```python
from build123d import *

# Parameters (mm, degrees)
SKETCH1_R           = 6.35
BOSS_EXTRUDE1_DEPTH = 254
SKETCH2_R           = 5.08
BOSS_EXTRUDE2_DEPTH = 203.2
SKETCH3_R           = 3.81
BOSS_EXTRUDE3_DEPTH = 152.4
SKETCH4_R           = 5.08
BOSS_EXTRUDE4_DEPTH = 7.62
FILLET1_R           = 2.54


with BuildPart() as part:
    # Sketch1 → Boss-Extrude1 (new body)
    with BuildSketch(Plane(origin=(0, 0, 0), x_dir=(1, 0, 0), z_dir=(0, 1, 0))):
        with Locations(Location((0, 0, 0), (0, 0, 270))):
            Circle(SKETCH1_R)
    extrude(amount=BOSS_EXTRUDE1_DEPTH)

    # Sketch2 → Boss-Extrude2 (add)
    with BuildSketch(Plane(origin=(0, 254, 0), x_dir=(1, 0, 0), z_dir=(0, 1, 0))):
        with Locations(Location((0, 0, 0), (0, 0, 270))):
            Circle(SKETCH2_R)
    extrude(amount=BOSS_EXTRUDE2_DEPTH)

    # Sketch3 → Boss-Extrude3 (add)
    with BuildSketch(Plane(origin=(0, 457.2, 0), x_dir=(1, 0, 0), z_dir=(0, 1, 0))):
        with Locations(Location((0, 0, 0), (0, 0, 90))):
            Circle(SKETCH3_R)
    extrude(amount=BOSS_EXTRUDE3_DEPTH)

    # Sketch4 → Boss-Extrude4 (add)
    with BuildSketch(Plane(origin=(0, 609.6, 0), x_dir=(1, 0, 0), z_dir=(0, 1, 0))):
        with Locations(Location((0, 0, 0), (0, 0, 270))):
            Circle(SKETCH4_R)
    extrude(amount=BOSS_EXTRUDE4_DEPTH)

    # Fillet1
    # the kernel refuses this fillet: 2.54 mm, written as the material it takes off along each edge
    with BuildSketch(Plane(origin=(0, 609.6, 0), x_dir=(0, 0, 1), z_dir=(-1, 0, 0))) as fillet1_piece_1:
        with BuildLine():
            CenterArc((2.54, 2.199704526), FILLET1_R, 300, 60)
            Line((3.81, 0), (3.8354, -0.043994091))
            ThreePointArc((3.8354, -0.043994091), (4.445, -0.0508), (5.08, -0.0508))
            Line((5.08, -0.0508), (5.1308, 0))
            Line((5.1308, 0), (5.1308, 2.199704526))
            Line((5.1308, 2.199704526), (5.08, 2.199704526))
        make_face()
    revolve(axis=Axis((0, 609.6, 0), (0, 1, 0)), mode=Mode.SUBTRACT)
    with BuildSketch(Plane(origin=(0, 617.22, 0), x_dir=(0, 0, 1), z_dir=(-1, 0, 0))) as fillet1_piece_2:
        with BuildLine():
            CenterArc((5.08 - FILLET1_R, -FILLET1_R), FILLET1_R, 0, 90)
            Line((5.08 - FILLET1_R, 0), (5.08 - FILLET1_R, FILLET1_R * 0.02))
            Line((5.08 - FILLET1_R, FILLET1_R * 0.02), (5.08 + FILLET1_R * 0.02, FILLET1_R * 0.02))
            Line((5.08 + FILLET1_R * 0.02, FILLET1_R * 0.02), (5.08 + FILLET1_R * 0.02, -FILLET1_R))
            Line((5.08 + FILLET1_R * 0.02, -FILLET1_R), (5.08, -FILLET1_R))
        make_face()
    revolve(axis=Axis((0, 617.22, 0), (0, 1, 0)), mode=Mode.SUBTRACT)


solid = part.part
```
The listing builds one solid part. Answer for the finished solid, in the listing's coordinates (mm). A direction names the side the tool comes from. Coordinates: 2 decimals unless noted, no trailing zeros. Write each loop counter-clockwise with the first axis right and the second up, starting at its lowest first coordinate (ties: lowest second). Pieces come first, ordered by that corner, then holes. Notation, with made-up numbers: (56, 31) - (75, 31) arc R33 ccw to (75, 66) - close; hole circle Ø2 at (42.5, 1.5). An arc over 180 degrees is marked (long way). Return JSON: item names as keys, results as strings. Group by question number.
1. Determine the mould class of faces 3 (the flat face through (4, 457.2, 1)), 4 (the flat face through (5, 254, 2)), 5 (the cylindrical face through (5.037, 354.178, -0.661)) for opening direction Y: released by +Y, released by -Y, zero draft, split by the parting line, or undercut.
2. A cutting plane is placed at A-A, the plane y = 39. Determine the outline of the cut face in (x, z), plus the area to 3 significant figures.
3. A cutting plane is placed at B-B, the plane y = 447. Determine the outline of the cut face in (x, z).
4. Given pin 1 (3 mm diameter, centred on x = 5, y = 486.5, fed in from -Z); pin 2 (5 mm diameter, centred on y = 461, z = -2.5, fed in from +X); pin 3 (1.5 mm diameter, centred on x = -4, y = 450, fed in from -Z); pin 4 (5 mm diameter, centred on x = 4, z = 3, fed in from -Y), each flat-ended and moving along its own axis, determine where each tip first touches the part or whether it passes through.
5. Straight lines are drawn through the part: L1, parallel to Y at x = -2.75, z = 5.5; L2, parallel to X at y = 187.5, z = -0.5; L3, parallel to Y at x = 2.75, z = 3. For each, find the intervals that lie inside material, in ascending order.
6. Which of the six approach directions +Z, -Z, +X, -X, +Y, -Y give full straight-line access (tool end or side, diameter ignored) to faces 1 (the cylindrical face through (5.037, 613.22, -0.661)), 2 (the cylindrical face through (-3.86, 125.22, -5.04))?
Ans:
{
 "1": {"face 3": "undercut", "face 4": "released by +Y", "face 5": "zero draft"},
 "2": {"outline": "circle Ø12.7 at (0, 0)", "area": "127 mm²"},
 "3": {"outline": "circle Ø10.16 at (0, 0)"},
 "4": {"pin 1": "z = -1.51", "pin 2": "x = 3.81", "pin 3": "z = -3.9", "pin 4": "y = 0"},
 "5": {"L1": "0 to 254", "L2": "-6.33 to 6.33", "L3": "0 to 457.2, 609.77 to 616.71"},
 "6": {"face 1": "+Y", "face 2": "+Y, -Y"}
}
